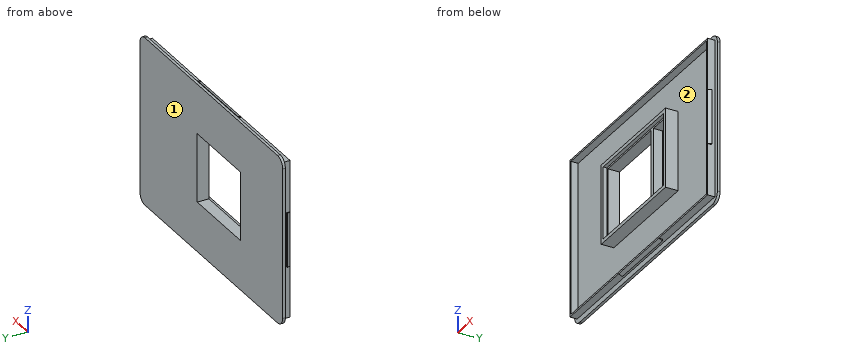
from build123d import *

# Parameters (mm, degrees)
SKETCH1_W                = 142
SKETCH1_H                = 93
BOSS_EXTRUDE1_DEPTH      = 1.5
SKETCH3_W                = 137
SKETCH3_H                = 87
SKETCH3_W_2              = 135
SKETCH3_H_2              = 85
EXTRUDE_THIN1_DEPTH      = 4
FILLET1_R                = 5
BOSS_EXTRUDE2_DEPTH      = 20
BOSS_EXTRUDE2_DEPTH_BACK = 20
BOSS_EXTRUDE3_DEPTH      = 15
BOSS_EXTRUDE3_DEPTH_BACK = 15
SKETCH6_W                = 58
SKETCH6_H                = 38
CUT_EXTRUDE2_DEPTH       = 10
SKETCH6_5_W              = 60
SKETCH6_5_H              = 40
SKETCH6_5_W_2            = 58
SKETCH6_5_H_2            = 38
BOSS_EXTRUDE4_DEPTH      = 5
SKETCH6_6_W              = 64
SKETCH6_6_H              = 44
SKETCH6_6_W_2            = 60
SKETCH6_6_H_2            = 40
BOSS_EXTRUDE5_DEPTH      = 7
SKETCH7_W                = 15
SKETCH7_H                = 38
BOSS_EXTRUDE6_DEPTH      = 1.5
BOSS_EXTRUDE7_REACH      = 67.5
SKETCH8_W                = 2.25753837
SKETCH8_H                = 5


with BuildPart() as part:
    # Sketch1 → Boss-Extrude1 (new body)
    with BuildSketch(Plane(origin=(0, 0, 0), x_dir=(1, 0, 0), z_dir=(0, 1, 0))):
        with Locations((68.5, 43.5)):
            Rectangle(SKETCH1_W, SKETCH1_H)
    extrude(amount=BOSS_EXTRUDE1_DEPTH)

    # Fillet1
    fillet1_edges = [part.edges().sort_by_distance(p)[0] for p in [
        (-2.5, 0.75, -90),
        (139.5, 0.75, -90),
        (139.5, 0.75, 3),
        (-2.5, 0.75, 3),
    ]]
    fillet(fillet1_edges, radius=FILLET1_R)

    # Sketch6 → Cut-Extrude2 (cut)
    with BuildSketch(Plane(origin=(0, 0, 0), x_dir=(-1, 0, 0), z_dir=(0, -1, 0))):
        with Locations((-68.5, 43.5)):
            Rectangle(SKETCH6_W, SKETCH6_H)
    extrude(amount=-CUT_EXTRUDE2_DEPTH, mode=Mode.SUBTRACT)


with BuildPart() as body_2:
    # Sketch3 → Extrude-Thin1 (new body)
    with BuildSketch(Plane(origin=(0, 0, 0), x_dir=(1, 0, 0), z_dir=(0, 1, 0))):
        with Locations((68.5, 43.5)):
            Rectangle(SKETCH3_W, SKETCH3_H)
        with Locations((68.5, 43.5)):
            Rectangle(SKETCH3_W_2, SKETCH3_H_2, mode=Mode.SUBTRACT)
    extrude(amount=-EXTRUDE_THIN1_DEPTH)

    # Sketch4 → Boss-Extrude2 (add, two sides)
    with BuildSketch(Plane(origin=(68.5, 0, 0), x_dir=(0, 0, -1), z_dir=(1, 0, 0))) as boss_extrude2_sk:
        Polygon((87, -2), (87, -4), (88, -2), align=None)
        Polygon((-1, -2), (0, -2), (0, -4), align=None)
    extrude(amount=BOSS_EXTRUDE2_DEPTH)
    extrude(boss_extrude2_sk.sketch, amount=-BOSS_EXTRUDE2_DEPTH_BACK)

    # Sketch5 → Boss-Extrude3 (add, two sides)
    with BuildSketch(Plane.XY.offset(-43.5)) as boss_extrude3_sk:
        Polygon((137, -2), (137, -4), (138, -2), align=None)
        Polygon((-1, -2), (0, -2), (0, -4), align=None)
    extrude(amount=BOSS_EXTRUDE3_DEPTH)
    extrude(boss_extrude3_sk.sketch, amount=-BOSS_EXTRUDE3_DEPTH_BACK)


    add(part.part)  # Boss-Extrude4 merges part
    # Sketch6_5 → Boss-Extrude4 (add)
    with BuildSketch(Plane(origin=(0, 0, 0), x_dir=(-1, 0, 0), z_dir=(0, -1, 0))):
        with Locations((-68.5, 43.5)):
            Rectangle(SKETCH6_5_W, SKETCH6_5_H)
        with Locations((-68.5, 43.5)):
            Rectangle(SKETCH6_5_W_2, SKETCH6_5_H_2, mode=Mode.SUBTRACT)
    extrude(amount=BOSS_EXTRUDE4_DEPTH)

    # Sketch6_6 → Boss-Extrude5 (add)
    with BuildSketch(Plane(origin=(0, 0, 0), x_dir=(-1, 0, 0), z_dir=(0, -1, 0))):
        with Locations((-68.5, 43.5)):
            Rectangle(SKETCH6_6_W, SKETCH6_6_H)
        with Locations((-68.5, 43.5)):
            Rectangle(SKETCH6_6_W_2, SKETCH6_6_H_2, mode=Mode.SUBTRACT)
    extrude(amount=BOSS_EXTRUDE5_DEPTH)

    # Sketch7 → Boss-Extrude6 (add)
    with BuildSketch(Plane(origin=(0, 1.5, 0), x_dir=(1, 0, 0), z_dir=(0, 1, 0))):
        with Locations((90, 43.5)):
            Rectangle(SKETCH7_W, SKETCH7_H)
    extrude(amount=-BOSS_EXTRUDE6_DEPTH)

    # Sketch8 → Boss-Extrude7 (add, up to next)
    with BuildSketch(Plane(origin=(0, 0, -24.5), x_dir=(-1, 0, 0), z_dir=(0, 0, -1)), mode=Mode.PRIVATE) as boss_extrude7_sk1:
        with Locations((-83.628769185, -2.5)):
            Rectangle(SKETCH8_W, SKETCH8_H)
    boss_extrude7_tool1 = extrude(boss_extrude7_sk1.sketch, amount=BOSS_EXTRUDE7_REACH, mode=Mode.PRIVATE) - body_2.part
    add(boss_extrude7_tool1.solids().sort_by_distance((83.628769, -2.5, -24.5))[0])


solid = body_2.part
Input: part model. Units: mm. Frame: model coordinates. Face numbers are marked on the shaded views. Coordinates: 2 decimals unless noted, no trailing zeros. Loops run counter-clockwise (first coordinate to the right, second up) from the corner with the lowest first, then second, coordinate; pieces in that order, holes last. Notation, with made-up numbers: (29.25, 79.5) -> (78.25, 79.5) arc R26 ccw to (78.25, 111.5) -> close; hole circle Ø6 at (-35, 85.5). An arc over 180 degrees is marked (long way). Write each question's results on one line, items separated by ' | '. Start each with the question number.
Q1. Pull-direction query (X, two-part tool) for the marked faces 1 and 2; classes: released by +X, released by -X, zero draft, split by the parting line, or undercut.
Q2. Section B-B, the plane x = 44. Return the cut outline in (y, z), plus the area to 4 significant figures.
Q3. Section C-C, the plane x = 22. Return the cut outline in (y, z).
Q4. Section A-A, the plane z = -26.5. Return the cut outline in (x, y), plus the area to 3 significant figures.
Q5. Section D-D, the plane z = -77. Return the cut outline in (x, y), plus the area to 3 significant figures.
Q6. Pin query (flat end, axial travel): pin 1 (1.5 mm diameter, centred on y = -3, z = -41.5, fed in from +X) (3 decimals); pin 2 (0.5 mm diameter, centred on y = -2.5, z = 0.5, fed in from +X); pin 3 (4 mm diameter, centred on y = -2.5, z = -32, fed in from +X). Return the tip coordinate at first contact, or that it passes through.
Q7. Ray query, line 1 (Z direction, x = 43, y = -3.25); line 2 (X direction, y = -0.25, z = -64); line 3 (X direction, y = -1.5, z = -40.5). Return the intervals inside material, ascending. Write a range as from..to.
Found:
1) face 1: zero draft | face 2: undercut
2) outline: (-7, -65.5) -> (0, -65.5) -> (0, -86) -> (-4, -86) -> (-4, -87) -> (0, -87) -> (0, -90) -> (1.5, -90) -> (1.5, -62.5) -> (-5, -62.5) -> (-5, -63.5) -> (-7, -63.5) -> close; (-7, -23.5) -> (-5, -23.5) -> (-5, -24.5) -> (1.5, -24.5) -> (1.5, 3) -> (0, 3) -> (0, 0) -> (-4, 0) -> (-4, -1) -> (0, -1) -> (0, -21.5) -> (-7, -21.5) -> close | area: 128.5 mm2
3) outline: (-4, -87) -> (0, -87) -> (0, -90) -> (1.5, -90) -> (1.5, 3) -> (0, 3) -> (0, 0) -> (-4, 0) -> (-4, -1) -> (0, -1) -> (0, -86) -> (-4, -86) -> close
4) outline: (-2.5, 0) -> (0, 0) -> (0, -4) -> (1, -4) -> (1, 0) -> (36.5, 0) -> (36.5, -7) -> (38.5, -7) -> (38.5, -5) -> (39.5, -5) -> (39.5, 1.5) -> (-2.5, 1.5) -> close; (82.5, -5) -> (84.76, -5) -> (84.76, 0) -> (97.5, 0) -> (97.5, -5) -> (98.5, -5) -> (98.5, -7) -> (100.5, -7) -> (100.5, 0) -> (136, 0) -> (136, -4) -> (137, -4) -> (137, 0) -> (139.5, 0) -> (139.5, 1.5) -> (82.5, 1.5) -> close | area: 206 mm2
5) outline: (-2.5, 0) -> (0, 0) -> (0, -4) -> (1, -4) -> (1, 0) -> (136, 0) -> (136, -4) -> (137, -4) -> (137, 0) -> (139.5, 0) -> (139.5, 1.5) -> (-2.5, 1.5) -> close | area: 221 mm2
6) pin 1: x = 137.875 | pin 2: x = 88.5 | pin 3: x = 138
7) line 1: -87..-86, -65.5..-62.5, -24.5..-21.5, -1..0 | line 2: 0..1, 36.5..100.5, 136..137 | line 3: 0..1, 36.5..39.5, 82.5..84.76, 97.5..100.5, 136..137
